CAD build for the part. Positions are in the model's coordinates, mm. Face numbers are marked on the shaded views. A direction names the side the tool comes from. Round coordinates to 2 decimals unless told otherwise and drop trailing zeros. Order: outer loops, then holes, each group sorted by start corner. A loop starts at its lowest first (then second) coordinate and runs counter-clockwise, first axis right, second up. Notation, with made-up numbers: (-28.5, 24) - (28.5, 24) arc R18 cw to (28.5, 38) - close; hole circle Ø4 at (47, 10.25). An arc over 180 degrees is marked (long way). Write item = value, one per line.
from build123d import *

# Parameters (mm, degrees)
F0_R      = 2.75
F0_R_2    = 11.5
F1_DEPTH  = 2
F3_DEPTH  = 29
F4_R      = 11.5
F4_R_2    = 2.75
F5_DEPTH  = 2
F0_R_3    = 9.5
F8_DEPTH  = 23
F9_DEPTH  = 7
F11_DEPTH = 19
F12_R     = 2.75
F13_DEPTH = 2


with BuildPart() as f1:
    # F0 (on Front) → F1 (new body)
    with BuildSketch(Plane.XZ):
        with BuildLine():
            Line((2.5, -40), (18.2350646454, -9.3665584597))
            ThreePointArc((18.2350646454, -9.3665584597), (0, 20.5), (-18.2350646454, -9.3665584597))
            Line((-18.2350646454, -9.3665584597), (-2.5, -40))
            Line((-2.5, -40), (2.5, -40))
        make_face()
        with Locations((0, -33)):
            Circle(F0_R, mode=Mode.SUBTRACT)
        Circle(F0_R_2, mode=Mode.SUBTRACT)
    extrude(amount=F1_DEPTH)

    # F0 (on Front) → F8 (join)
    with BuildSketch(Plane.XZ):
        Circle(F0_R_2)
        Circle(F0_R_3, mode=Mode.SUBTRACT)
    extrude(amount=F8_DEPTH)

    # F0 (on Front) → F9 (join)
    with BuildSketch(Plane.XZ):
        with Locations((0, -33)):
            Circle(F0_R)
    extrude(amount=F9_DEPTH)

    # F10 (on face) → F11 (cut)
    with BuildSketch(Plane.XZ.offset(23)):
        with BuildLine():
            Line((-8.129197368, -4.9159078665), (-10.3963382904, -4.9159078665))
            ThreePointArc((-10.3963382904, -4.9159078665), (0, -11.5), (10.3963382904, -4.9159078665))
            Line((10.3963382904, -4.9159078665), (8.129197368, -4.9159078665))
            ThreePointArc((8.129197368, -4.9159078665), (0, -9.5), (-8.129197368, -4.9159078665))
        make_face()
    extrude(amount=-F11_DEPTH, mode=Mode.SUBTRACT)

    # F12 (on face) → F13 (join)
    with BuildSketch(Plane.XZ.offset(23)):
        with BuildLine():
            Line((8.129197368, -4.9159078665), (10.3963382904, -4.9159078665))
            ThreePointArc((10.3963382904, -4.9159078665), (11.2206927224, -2.5191377156), (11.5, 0))
            ThreePointArc((11.5, 0), (-2.5191377156, 11.2206927224), (-10.3963382904, -4.9159078665))
            Line((-10.3963382904, -4.9159078665), (-8.129197368, -4.9159078665))
            ThreePointArc((-8.129197368, -4.9159078665), (-2.5517273565, 9.15088452), (9.5, 0))
            ThreePointArc((9.5, 0), (9.15088452, -2.5517273565), (8.129197368, -4.9159078665))
        make_face()
        with BuildLine():
            Line((-8.129197368, -4.9159078665), (8.129197368, -4.9159078665))
            ThreePointArc((8.129197368, -4.9159078665), (9.15088452, -2.5517273565), (9.5, 0))
            ThreePointArc((9.5, 0), (-2.5517273565, 9.15088452), (-8.129197368, -4.9159078665))
        make_face()
        Circle(F12_R, mode=Mode.SUBTRACT)
    extrude(amount=F13_DEPTH)


with BuildPart() as f3:
    # F2 (on face) → F3 (new body)
    with BuildSketch(Plane(origin=(0, 0, 0), x_dir=(-1, 0, 0), z_dir=(0, 1, 0))):
        with BuildLine():
            ThreePointArc((0, 11.5), (-8.1317279836, 8.1317279836), (-11.5, 0))
            ThreePointArc((-11.5, 0), (-11.2103927734, -2.5645845405), (-10.3561575886, -5))
            Line((-10.3561575886, -5), (-8.6602540378, -5))
            ThreePointArc((-8.6602540378, -5), (0, 10), (8.6602540378, -5))
            Line((8.6602540378, -5), (10.3561575886, -5))
            ThreePointArc((10.3561575886, -5), (11.2103927734, -2.5645845405), (11.5, 0))
            ThreePointArc((11.5, 0), (8.1317279836, 8.1317279836), (0, 11.5))
        make_face()
    extrude(amount=F3_DEPTH)


with BuildPart() as f5:
    # F4 (on Front) → F5 (new body)
    with BuildSketch(Plane.XZ):
        Circle(F4_R)
        Circle(F4_R_2, mode=Mode.SUBTRACT)
    extrude(amount=F5_DEPTH)


solid = f1.part
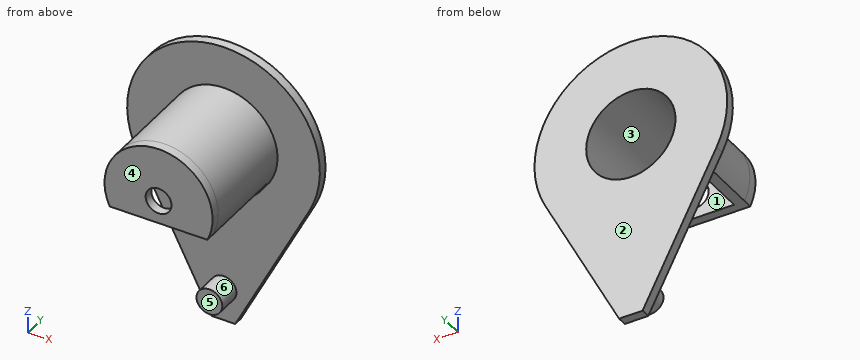
(1) Probe line 1 along X through (y, z) = (-8, 0); line 2 along Y through (x, z) = (-8, -18.5); line 3 along Z through (x, y) = (0, -9.75). List the from-to ranges inside material, lowest first.
Solved:
line_1 = -11.5 to -9.5, 9.5 to 11.5
line_2 = -2 to 0
line_3 = 9.5 to 11.5
(2) Pull direction Z, two halves, no side cores. Call the marked faces 1, 2 and 3: released by +Z, released by -Z, zero draft, split by the parting line, or undercut.
Solved:
face_1 = undercut
face_2 = zero draft
face_3 = undercut
(3) Band-saw the part on D-D on z = -8. List the corners of the cut face in (x, y), plus the area to 3 significant figures.
Solved:
outline = (-18.87, -2) - (-8.26, -2) - (-8.26, -4) - (-5.12, -4) - (-5.12, 0) - (-18.87, 0) - close; (5.12, -4) - (8.26, -4) - (8.26, -2) - (18.87, -2) - (18.87, 0) - (5.12, 0) - close
area = 67.6 mm²
(4) Band-saw the part on B-B on y = -2.75. List the corners of the cut face in (x, z), plus the area to 3 significant figures.
Solved:
outline = circle Ø23 at (0, 0); circle Ø5.5 at (0, -33); hole circle Ø19 at (0, 0)
area = 156 mm²
(5) Tool access for the marked faces 4, 5 and 6: list every direction of +Z, -Z, +X, -X, +Y, -Y with a clear straight run to the whole face (end or side of a thin tool).
Solved:
face_4 = +Z, -Z, +X, -X, -Y
face_5 = -Z, +X, -X, -Y
face_6 = -Y
(6) Drop flat-ended pins along their axis: pin 1 (7 mm diameter, centred on x = -1.5, z = -1, fed in from +Y); pin 2 (6 mm diameter, centred on x = -1, y = -14.5, fed in from -Z); pin 3 (8 mm diameter, centred on x = -1.5, y = -22, fed in from +Z). Give the stop position or say it passes through.
Solved:
pin_1 = -23
pin_2 = 8.62
pin_3 = 11.5
(7) Band-saw the part on C-C on x = -4.5. List the corners of the cut face in (y, z), plus the area to 3 significant figures.
Solved:
outline = (-25, -4.92) - (-23, -4.92) - (-23, 8.37) - (0, 8.37) - (0, 20) - (-2, 20) - (-2, 10.58) - (-25, 10.58) - close; (-4, -10.58) - (-2, -10.58) - (-2, -36.11) - (0, -36.11) - (0, -8.37) - (-4, -8.37) - close
area = 161 mm²
(8) Band-saw the part on A-A on x = 0. List the corners of the cut face in (y, z), plus the area to 3 significant figures.
Solved:
outline = (-25, -4.92) - (-23, -4.92) - (-23, -2.75) - (-25, -2.75) - close; (-25, 2.75) - (-23, 2.75) - (-23, 9.5) - (0, 9.5) - (0, 20.5) - (-2, 20.5) - (-2, 11.5) - (-25, 11.5) - close; (-7, -35.75) - (-2, -35.75) - (-2, -40) - (0, -40) - (0, -9.5) - (-4, -9.5) - (-4, -11.5) - (-2, -11.5) - (-2, -30.25) - (-7, -30.25) - close
area = 178 mm²
